```python
from build123d import *

# Parameters (mm, degrees)
EXTRUDE_THIN1_DEPTH = 381
FILLET1_R           = 0.889


with BuildPart() as part:
    # Sketch1 → Extrude-Thin1 (new body)
    with BuildSketch(Plane.XY):
        with BuildLine():
            Line((0, 27.78125), (0, 36.2966))
            Line((0, 36.2966), (5.4483, 36.2966))
            ThreePointArc((5.4483, 36.2966), (6.35, 37.1983), (5.4483, 38.1))
            Line((5.4483, 38.1), (-7.9375, 38.1))
            ThreePointArc((-7.9375, 38.1), (-11.305096045, 36.705096045), (-12.7, 33.3375))
            Line((-12.7, 33.3375), (-12.7, 22.225))
            ThreePointArc((-12.7, 22.225), (-8.097870067, 18.744005193), (-6.35, 13.244743879))
            Line((-6.35, 13.244743879), (-6.35, 0))
            Line((-6.35, 0), (0, 0))
            Line((0, 0), (0, 10.31875))
            Line((0, 10.31875), (-0.889, 10.31875))
            Line((-0.889, 10.31875), (-0.889, 0.889))
            Line((-0.889, 0.889), (-5.461, 0.889))
            Line((-5.461, 0.889), (-5.461, 13.244743879))
            ThreePointArc((-5.461, 13.244743879), (-7.192434365, 18.994913442), (-11.811, 22.833033612))
            Line((-11.811, 22.833033612), (-11.811, 33.3375))
            ThreePointArc((-11.811, 33.3375), (-10.676478117, 36.076478117), (-7.9375, 37.211))
            Line((-7.9375, 37.211), (5.4483, 37.211))
            ThreePointArc((5.4483, 37.211), (5.461, 37.1983), (5.4483, 37.1856))
            Line((5.4483, 37.1856), (-0.889, 37.1856))
            Line((-0.889, 37.1856), (-0.889, 27.78125))
            Line((-0.889, 27.78125), (0, 27.78125))
        make_face()
    extrude(amount=-EXTRUDE_THIN1_DEPTH)

    # Fillet1
    fillet1_edges = [part.edges().sort_by_distance(p)[0] for p in [
        (0, 0, -190.5),
        (-6.35, 0, -190.5),
        (-12.7, 22.225, -190.5),
        (-0.889, 37.1856, -190.5),
    ]]
    fillet(fillet1_edges, radius=FILLET1_R)


solid = part.part
```
Source: CAD feature listing. Evaluate the final solid. Frame: model axes, mm. A direction names the side the tool comes from. Round coordinates to 2 decimals unless told otherwise and drop trailing zeros. Loops run counter-clockwise (first coordinate to the right, second up) from the corner with the lowest first, then second, coordinate; pieces in that order, holes last.
1. Mould query, pull axis Z, two halves, no side actions, for faces 5 (the flat face through (-0.889, 6, -188)), 6 (the flat face through (-8.9, 20.6, 0)), 7 (the flat face through (-1, 37.211, -188)), 8 (the flat face through (-8.9, 20.6, -381)). Classes: released by +Z, released by -Z, zero draft, split by the parting line, or undercut.
2. Section query A-A on y = 6. Output: boundary loops of the cut face in (x, z).
3. Ray query, L1, parallel to X at y = 3.5, z = -150; L2, parallel to Y at x = -1.25, z = -117.5; L3, parallel to Y at x = -8, z = -355. Return the intervals inside material, ascending.
4. Access query for faces 1 (the flat face through (-5.461, 7, -188)), 2 (the cylindrical face through (-7.146, 18.924, -187.833)), 3 (the flat face through (0, 6, -188)), 4 (the flat face through (-6.35, 7, -188)). Directions: +Z, -Z, +X, -X, +Y, -Y. A direction counts if a zero-diameter tool reaches every point of the face in a straight line with its end or side. Return the directions, or none.
5. Contact query for flat-ended pins moving along their axis: pin 1 (8.5 mm diameter, centred on y = 29.5, z = -126.5, fed in from +X); pin 2 (4 mm diameter, centred on x = -9.5, z = -121, fed in from -Y); pin 3 (2 mm diameter, centred on y = 19.5, z = -298.5, fed in from +X); pin 4 (1.5 mm diameter, centred on x = 1, y = 30, fed in from +Z). Output: stop coordinate, or through.
Answers below:
1. face 5: zero draft
1. face 6: released by +Z
1. face 7: undercut
1. face 8: released by -Z
2. outline: (-6.35, -381) - (-5.46, -381) - (-5.46, 0) - (-6.35, 0) - close; (-0.89, -381) - (0, -381) - (0, 0) - (-0.89, 0) - close
3. L1: x = -6.35 to -5.46, -0.89 to 0
3. L2: y = 0 to 0.89, 37.21 to 38.1
3. L3: y = 18.6 to 20.06, 37.21 to 38.1
4. face 1: +Z, -Z
4. face 2: +Z, -Z, +X
4. face 3: +Z, -Z, +X, -Y
4. face 4: +Z, -Z, -X, -Y
5. pin 1: stops at x = 0
5. pin 2: stops at y = 17.78
5. pin 3: stops at x = -6.88
5. pin 4: passes through
